```python
from build123d import *

# Parameters (mm, degrees)
EXTRUDE_1_DEPTH     = 6
SKETCH_2_R          = 5.75
EXTRUDE_2_DEPTH     = 12
SKETCH_3_R          = 2.5
CUT_EXTRUDE_1_DEPTH = 29
SKETCH_5_R          = 1.65
CUT_EXTRUDE_2_DEPTH = 3.5
FILLET_2_R          = 0.1


with BuildPart() as part:
    # 草图1 → 凸台-拉伸1 (new body)
    with BuildSketch(Plane(origin=(0, 0, 0), x_dir=(1, 0, 0), z_dir=(0, 1, 0))):
        Polygon((-3.5, -6.062177826), (3.5, -6.062177826), (7, 0), (3.5, 6.062177826), (-3.5, 6.062177826), (-7, 0), align=None)
    extrude(amount=EXTRUDE_1_DEPTH)

    # 草图2 → 凸台-拉伸2 (add)
    with BuildSketch(Plane.XZ):
        Circle(SKETCH_2_R)
    extrude(amount=EXTRUDE_2_DEPTH)

    # 草图3 → 切除-拉伸1 (cut)
    with BuildSketch(Plane(origin=(0, 6, 0), x_dir=(1, 0, 0), z_dir=(0, 1, 0))):
        Circle(SKETCH_3_R)
    extrude(amount=-CUT_EXTRUDE_1_DEPTH, mode=Mode.SUBTRACT)

    # 草图4 → 切除-旋转1 (revolve, cut)
    with BuildSketch(Plane.XY):
        with BuildLine():
            Line((-7, 0), (-6.600189391, 0))
            ThreePointArc((-6.600189391, 0), (-6.822809169, 0.548107865), (-7, 1.112541391))
            Line((-7, 1.112541391), (-7, 0))
        make_face()
        with BuildLine():
            Line((-7, 6), (-7, 4.887458609))
            ThreePointArc((-7, 4.887458609), (-6.822809169, 5.451892135), (-6.600189391, 6))
            Line((-6.600189391, 6), (-7, 6))
        make_face()
    revolve(axis=Axis((0, -23, 0), (0, 1, 0)), mode=Mode.SUBTRACT)

    # 草图5 → 切除-拉伸2 (cut, symmetric)
    with BuildSketch(Plane(origin=(1.75, 0, 3.031088913), x_dir=(0.866025404, 0, -0.5), z_dir=(0.5, 0, 0.866025404))):
        with Locations((0, -9)):
            Circle(SKETCH_5_R)
    extrude(amount=CUT_EXTRUDE_2_DEPTH, both=True, mode=Mode.SUBTRACT)

    # 圆角2
    fillet_2_edges = [part.edges().sort_by_distance(p)[0] for p in [
        (-5.75, -12, 0),
        (-2.5, -12, 0),
    ]]
    fillet(fillet_2_edges, radius=FILLET_2_R)


solid = part.part
```
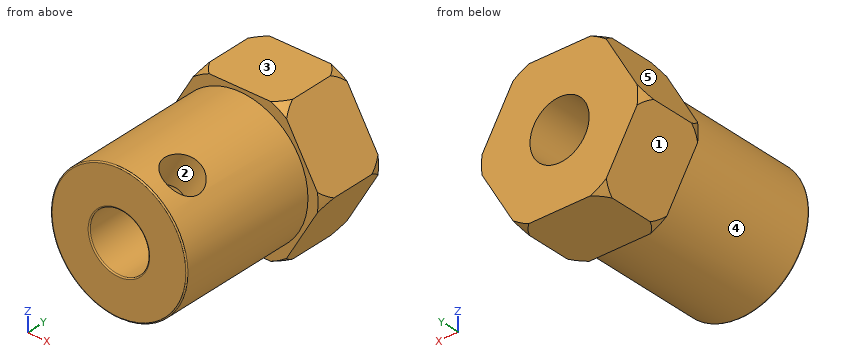
Verification items for the finished model (mm, model axes). Face numbers are marked on the shaded views. A direction names the side the tool comes from. Coordinates: 2 decimals unless noted, no trailing zeros. Loops run counter-clockwise (first coordinate to the right, second up) from the corner with the lowest first, then second, coordinate; pieces in that order, holes last. Notation, with made-up numbers: (-4, 60.25) -> (0, 60.25) arc R31 ccw to (0, 91.25) -> close; hole circle Ø1 at (-8.5, 1.25). An arc over 180 degrees is marked (long way). Answer in a Markdown table with one row per item. Add a question column.
1. Access from +Z, -Z, +X, -X, +Y, -Y to the whole of each face (thin tool, end or side, straight path). Record for the marked faces 4 and 5.
2. Section check A-A, the plane y = -6. Enter the section's corners in (x, z), then the cut area to 3 significant figures.
3. Draft check along X on the marked faces 1, 2 and 3. Enter one of: +X half, -X half, draft (parallel to the pull), parting line (faces both ways), or undercut.
4. Depth check by flat-ended pin: P1, Ø6, axis at x = 0, z = 0, coming from the +Y side; P2, Ø3, axis at y = -3.5, z = -3, coming from the -X side; P3, Ø1, axis at y = -5.5, z = -1.5, coming from the -X side; P4, Ø8, axis at x = 1.5, y = -6.5, coming from the -Z side. Enter the tip coordinate at first touch or a pass-through.
5. Material ranges on probe 1 along Z at (x, y) = (0, -2.5); probe 2 along Z at (x, y) = (0, 1.25); probe 3 along Y at (x, z) = (2.25, 1.25), recorded low to high. Write a range as [from, to].
Derived:
| question | item | result |
|---|---|---|
| 1 | face 4 | -Y |
| 1 | face 5 | +Z, -X, +Y, -Y |
| 2 | outline | circle Ø11.5 at (0, 0); hole circle Ø5 at (0, 0) |
| 2 | area | 84.2 mm² |
| 3 | face 1 | -X half |
| 3 | face 2 | undercut |
| 3 | face 3 | draft |
| 4 | P1 | stops at y = 6 |
| 4 | P2 | stops at x = -5.55 |
| 4 | P3 | stops at x = -5.66 |
| 4 | P4 | stops at z = -5.75 |
| 5 | probe 1 | z = [-5.75, -2.5], [2.5, 5.75] |
| 5 | probe 2 | z = [-6.06, -2.5], [2.5, 6.06] |
| 5 | probe 3 | y = [-12, -9.99], [-8.01, 6] |
